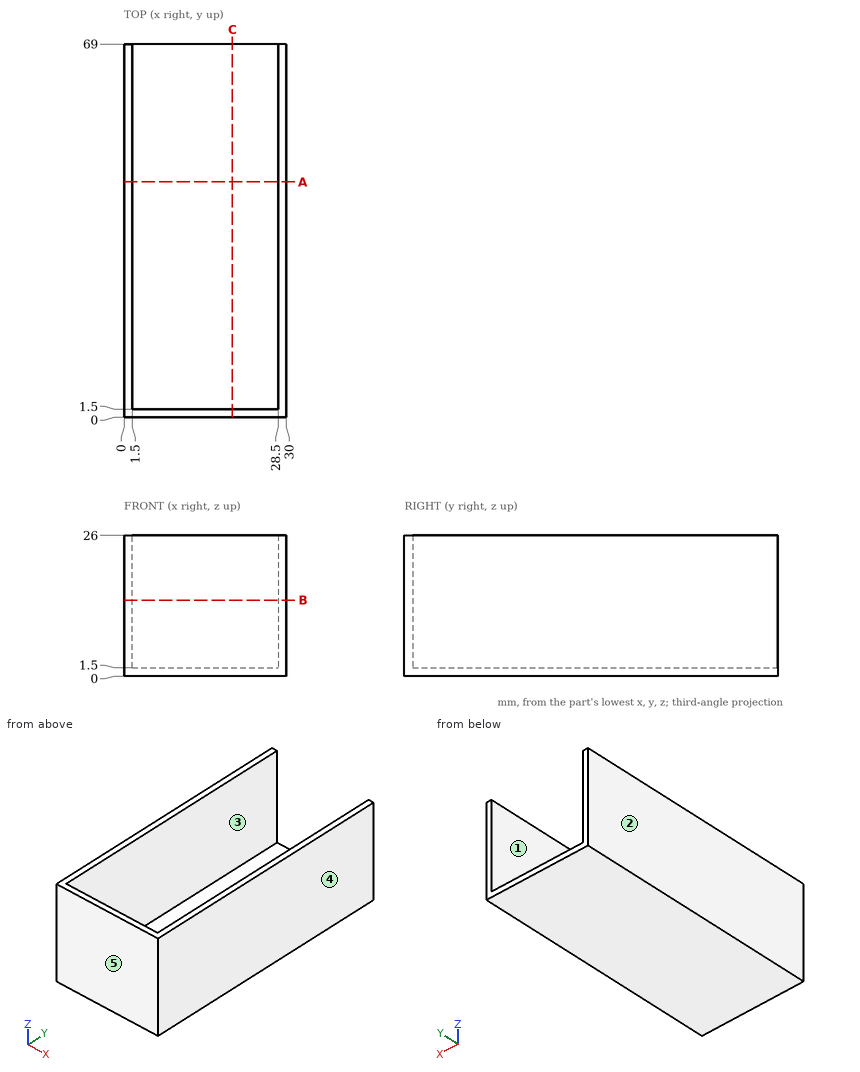
For this review, use the dimensioned drawing (mm, ordinates from the lowest corner) and the shaded views. A direction names the side the tool comes from. Give positions to 0.01 mm unless a question says otherwise; leave off trailing zeros. Order: outer loops, then holes, each group sorted by start corner. A loop starts at its lowest first (then second) coordinate and runs counter-clockwise, first axis right, second up. Notation, with made-up numbers: (25.5, 72.5) - (72.5, 72.5) arc R21 ccw to (72.5, 85.5) - close; hole circle Ø2 at (-19.75, -12). An arc over 180 degrees is marked (long way). Use CSV: the item, a comma, the result in double quotes. Start each with the question number.
Q1. Take a section at A-A (y = 43.5). State the section outline as (x, z) points, and give its area (4 significant figures).
Q2. Draft analysis for pull direction X (two halves, no side actions). For the marked faces 3, 4 and 5, state which applies: pulls with the +X half, pulls with the -X half, needs draft (parallel to the pull), parting line crosses it, or undercut.
Q3. For P1, Ø1.5, axis at x = 17, z = 16, coming from the +Y side, flat-tipped, find the tip position at first contact; note if it passes through.
Q4. Take a section at B-B (z = 14). State the section outline as (x, y) points, and give its area (4 significant figures).
Q5. For line 1 (X direction, y = 13, z = 8.25); line 2 (Y direction, x = 26.5, z = 16), list the stretches that pass through material, from the lowest coordinate up.
Q6. Machinability: for the marked faces 1 and 2, which of the approach directions +Z, -Z, +X, -X, +Y, -Y give a long, thin tool a straight path to every point of the face, cutting with its end or side? Answer none if there is none.
Q7. Take a section at C-C (x = 20). State the section outline as (y, z) points, and give its area (3 significant figures).
Calculated:
1,outline,"(0, 0) - (30, 0) - (30, 26) - (28.5, 26) - (28.5, 1.5) - (1.5, 1.5) - (1.5, 26) - (0, 26) - close"
1,area,"118.5 mm²"
2,face 3,"undercut"
2,face 4,"pulls with the +X half"
2,face 5,"needs draft"
3,P1,"stops at y = 1.5"
4,outline,"(0, 0) - (30, 0) - (30, 69) - (28.5, 69) - (28.5, 1.5) - (1.5, 1.5) - (1.5, 69) - (0, 69) - close"
4,area,"247.5 mm²"
5,line 1,"x = 0 to 1.5, 28.5 to 30"
5,line 2,"y = 0 to 1.5"
6,face 1,"+Z, +Y"
6,face 2,"+Z, -Z, -X, +Y, -Y"
7,outline,"(0, 0) - (69, 0) - (69, 1.5) - (1.5, 1.5) - (1.5, 26) - (0, 26) - close"
7,area,"140 mm²"
